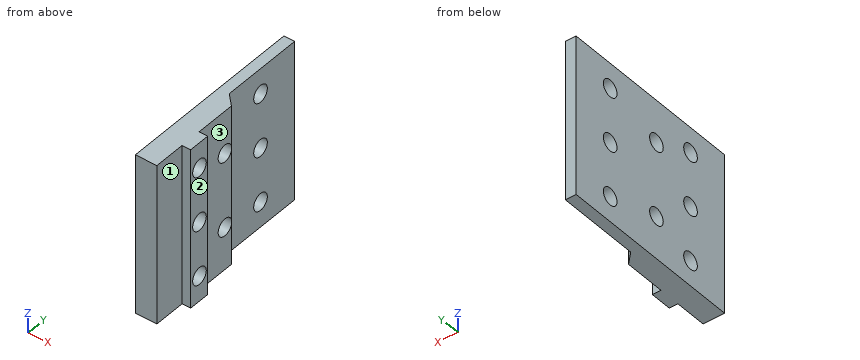
```python
from build123d import *

# Parameters (mm, degrees)
BOSS_EXTRUDE1_DEPTH = 47.625
SKETCH2_R           = 2.54
CUT_EXTRUDE1_DEPTH  = 9.89


with BuildPart() as part:
    # Sketch1 → Boss-Extrude1 (new body)
    with BuildSketch(Plane.XY):
        Polygon((0, 0), (0, 55.3466), (3.175, 55.3466), (3.175, 30.988), (6.35, 27.813), (6.35, 15.748), (8.89, 15.748), (8.89, 9.398), (6.35, 9.398), (6.35, 0), align=None)
    extrude(amount=BOSS_EXTRUDE1_DEPTH)

    # Sketch2 → Cut-Extrude1 (cut, through all)
    with BuildSketch(Plane.ZY):
        with Locations((40.0685, 12.7)):
            Circle(SKETCH2_R)
        with Locations((7.5565, 12.7)):
            Circle(SKETCH2_R)
        with Locations((12.7, 25.4)):
            Circle(SKETCH2_R)
        with Locations((34.925, 25.4)):
            Circle(SKETCH2_R)
        with Locations((7.5565, 42.6466)):
            Circle(SKETCH2_R)
        with Locations((40.0685, 42.6466)):
            Circle(SKETCH2_R)
        with Locations((23.8125, 12.7)):
            Circle(SKETCH2_R)
        with Locations((23.8125, 42.6466)):
            Circle(SKETCH2_R)
    extrude(amount=-CUT_EXTRUDE1_DEPTH, mode=Mode.SUBTRACT)


solid = part.part
```
Read the model definition and answer for the solid it produces. Units are mm, in the model's axes. Face numbers are marked on the shaded views. A direction names the side the tool comes from. Give positions to 0.01 mm unless a question says otherwise; leave off trailing zeros. Write each loop counter-clockwise with the first axis right and the second up, starting at its lowest first coordinate (ties: lowest second). Pieces come first, ordered by that corner, then holes. Notation, with made-up numbers: (-4.5, 73.25) -> (3.5, 73.25) arc R11 cw to (3.5, 92.25) -> close; hole circle Ø9 at (76.5, -18). An arc over 180 degrees is marked (long way). Answer as a JSON object with one key per item and string values.
1) A tool of negligible diameter and unlimited length cuts with its end or side. For the marked faces 1, 2 and 3, from which of +Z, -Z, +X, -X, +Y, -Y can it reach the whole face along a straight path? Write none if from no direction.
Findings below:
{"face 1": "+Z, -Z, +X, -Y", "face 2": "+Z, -Z, +X, +Y, -Y", "face 3": "+Z, -Z, +X, +Y"}
2) Section D-D on y = 25.4 is taken. Write down the section's boundary in (x, z) (3 decimals).
Findings below:
{"outline": "(0, 0) -> (6.35, 0) -> (6.35, 10.16) -> (0, 10.16) -> close; (0, 15.24) -> (6.35, 15.24) -> (6.35, 32.385) -> (0, 32.385) -> close; (0, 37.465) -> (6.35, 37.465) -> (6.35, 47.625) -> (0, 47.625) -> close"}
3) Section B-B on x = 7 is taken. Write down the section's boundary in (y, z) (1 decimal), then the cut area to 3 significant figures.
Findings below:
{"outline": "(9.4, 0) -> (15.7, 0) -> (15.7, 47.6) -> (9.4, 47.6) -> close; hole circle Ø5.1 at (12.7, 7.6); hole circle Ø5.1 at (12.7, 23.8); hole circle Ø5.1 at (12.7, 40.1)", "area": "242 mm^2"}
4) Section C-C on z = 39 is taken. Write down the section's boundary in (x, y) (3 decimals), then the cut area to 3 significant figures.
Findings below:
{"outline": "(0, 0) -> (6.35, 0) -> (6.35, 9.398) -> (8.89, 9.398) -> (8.89, 10.396) -> (0, 10.396) -> close; (0, 15.004) -> (8.89, 15.004) -> (8.89, 15.748) -> (6.35, 15.748) -> (6.35, 27.813) -> (3.175, 30.988) -> (3.175, 40.342) -> (0, 40.342) -> close; (0, 44.951) -> (3.175, 44.951) -> (3.175, 55.347) -> (0, 55.347) -> close", "area": "230 mm^2"}
5) Section A-A on y = 12.7 is taken. Write down the section's boundary in (x, z) (1 decimal).
Findings below:
{"outline": "(0, 0) -> (8.9, 0) -> (8.9, 5) -> (0, 5) -> close; (0, 10.1) -> (8.9, 10.1) -> (8.9, 21.3) -> (0, 21.3) -> close; (0, 26.4) -> (8.9, 26.4) -> (8.9, 37.5) -> (0, 37.5) -> close; (0, 42.6) -> (8.9, 42.6) -> (8.9, 47.6) -> (0, 47.6) -> close"}
6) Flat-ended cylindrical pins translate along their axes: pin 1 Ø0.8 at (x, z) = (8, 14.5) entering from -Y; pin 2 Ø6.5 at (y, z) = (42.65, 7.56) entering from +X (3 decimals); pin 3 Ø3.5 at (y, z) = (22.5, 31) entering from +X; pin 4 Ø3 at (y, z) = (12.7, 40.07) entering from -X. Find the tip coordinate at first contact, or state that the pin passes through.
Findings below:
{"pin 1": "stops at y = 9.4", "pin 2": "stops at x = 3.175", "pin 3": "stops at x = 6.35", "pin 4": "passes through"}
7) Straight lines are drawn through the part: probe 1 along Z at (x, y) = (6.5, 12.5) (3 decimals); probe 2 along Z at (x, y) = (3, 25.4) (3 decimals); probe 3 along Y at (x, z) = (8.25, 40). For each, find the intervals that lie inside material, in ascending order. Write a range as from..to.
Findings below:
{"probe 1": "z = 0..5.024, 10.089..21.28, 26.345..37.536, 42.601..47.625", "probe 2": "z = 0..10.16, 15.24..32.385, 37.465..47.625", "probe 3": "y = 9.4..10.16, 15.24..15.75"}
